Input: part model. Units: mm. Frame: model coordinates. Face numbers are marked on the shaded views. A direction names the side the tool comes from. Round coordinates to 2 decimals unless told otherwise and drop trailing zeros. Loops run counter-clockwise (first coordinate to the right, second up) from the corner with the lowest first, then second, coordinate; pieces in that order, holes last.
1) Ray query, line 1 along Y through (x, z) = (-87, 2); line 2 along Z through (x, y) = (-31.5, -7.5); line 3 along Z through (x, y) = (-36.5, -10). Return the intervals inside material, ascending.
2) Section A-A, the plane z = 4. Return loops of the section in (x, y), and give its area (3 significant figures).
3) Section B-B, the plane y = 3. Return loops of the section in (x, z).
4) Draft query along Z for the marked faces 1, 2 and 3. Return one class per face: pulls with the +Z half, pulls with the -Z half, needs draft (parallel to the pull), parting line crosses it, or undercut.
5) Access query for the marked faces 4 and 5. Directions: +Z, -Z, +X, -X, +Y, -Y. A direction counts if a zero-diameter tool reaches every point of the face in a straight line with its end or side. Return the directions, or none.
6) Section C-C, the plane x = 2. Return loops of the section in (y, z), and give its area (3 significant figures).
7) First-contact query: pin 1 (10 mm diameter, centred on y = 5, z = -15, fed in from +X); pin 2 (12 mm diameter, centred on y = 6.5, z = 3.5, fed in from -X). Flat tips, straight axial feed; report the tip coordinate or a pass-through.
from build123d import *

# Parameters (mm, degrees)
F0_W     = 261.9375
F0_H     = 50.8
F1_DEPTH = 12.7
F2_T     = -2.54
F4_DEPTH = 50.801
F5_R     = 1.27
F6_R     = 2.54


with BuildPart() as f1:
    # F0 (on Front) → F1 (new body, symmetric)
    with BuildSketch(Plane.XZ):
        Rectangle(F0_W, F0_H)
    extrude(amount=F1_DEPTH, both=True)

    # F2
    f2_openings = [f1.faces().sort_by_distance(p)[0] for p in [
        (-130.96875, 0, 0),
        (130.96875, 0, 0),
    ]]
    offset(amount=F2_T, openings=f2_openings)

    # F3 (on face) → F4 (cut, through all)
    with BuildSketch(Plane.XY.offset(25.4)):
        Polygon((-86.9746594878, -12.7), (-130.96875, 12.7), (-130.96875, -12.7), align=None)
    extrude(amount=-F4_DEPTH, mode=Mode.SUBTRACT)

    # F5
    f5_edges = [f1.edges().sort_by_distance(p)[0] for p in [
        (2.199705, 10.16, -22.86),
        (2.199705, 10.16, 22.86),
        (19.797341, -10.16, 22.86),
        (19.797341, -10.16, -22.86),
    ]]
    fillet(f5_edges, radius=F5_R)

    # F6
    f6_edges = [f1.edges().sort_by_distance(p)[0] for p in [
        (21.997045, -12.7, 25.4),
        (0, 12.7, 25.4),
        (0, 12.7, -25.4),
        (21.997045, -12.7, -25.4),
    ]]
    fillet(f6_edges, radius=F6_R)


solid = f1.part
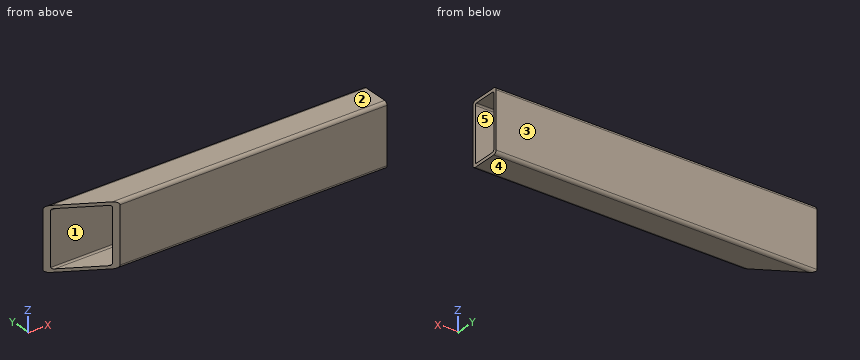
Final values:
1. line 1: y = -12.69 to -10.16, 10.16 to 12.7
1. line 2: z = -25.4 to -22.86, 22.86 to 25.4
1. line 3: z = -25.4 to -22.21, 22.21 to 25.4
2. outline: (-130.97, 12.7) - (-126.57, 10.16) - (130.97, 10.16) - (130.97, 12.7) - close; (-91.37, -10.16) - (-86.97, -12.7) - (130.97, -12.7) - (130.97, -10.16) - close
2. area: 1,220 mm2
3. outline: (-114.17, -25.4) - (130.97, -25.4) - (130.97, -22.86) - (-114.17, -22.86) - close; (-114.17, 22.86) - (130.97, 22.86) - (130.97, 25.4) - (-114.17, 25.4) - close
4. face 1: undercut
4. face 2: pulls with the +Z half
4. face 3: needs draft
5. face 4: -Z, +X, -X, +Y, -Y
5. face 5: +X, -X
6. outline: (-12.7, -22.86) arc R2.54 ccw to (-10.16, -25.4) - (10.16, -25.4) arc R2.54 ccw to (12.7, -22.86) - (12.7, 22.86) arc R2.54 ccw to (10.16, 25.4) - (-10.16, 25.4) arc R2.54 ccw to (-12.7, 22.86) - close; hole (-10.16, -21.59) arc R1.27 ccw to (-8.89, -22.86) - (8.89, -22.86) arc R1.27 ccw to (10.16, -21.59) - (10.16, 21.59) arc R1.27 ccw to (8.89, 22.86) - (-8.89, 22.86) arc R1.27 ccw to (-10.16, 21.59) - close
6. area: 357 mm2
7. pin 1: passes through
7. pin 2: stops at x = -130.62
